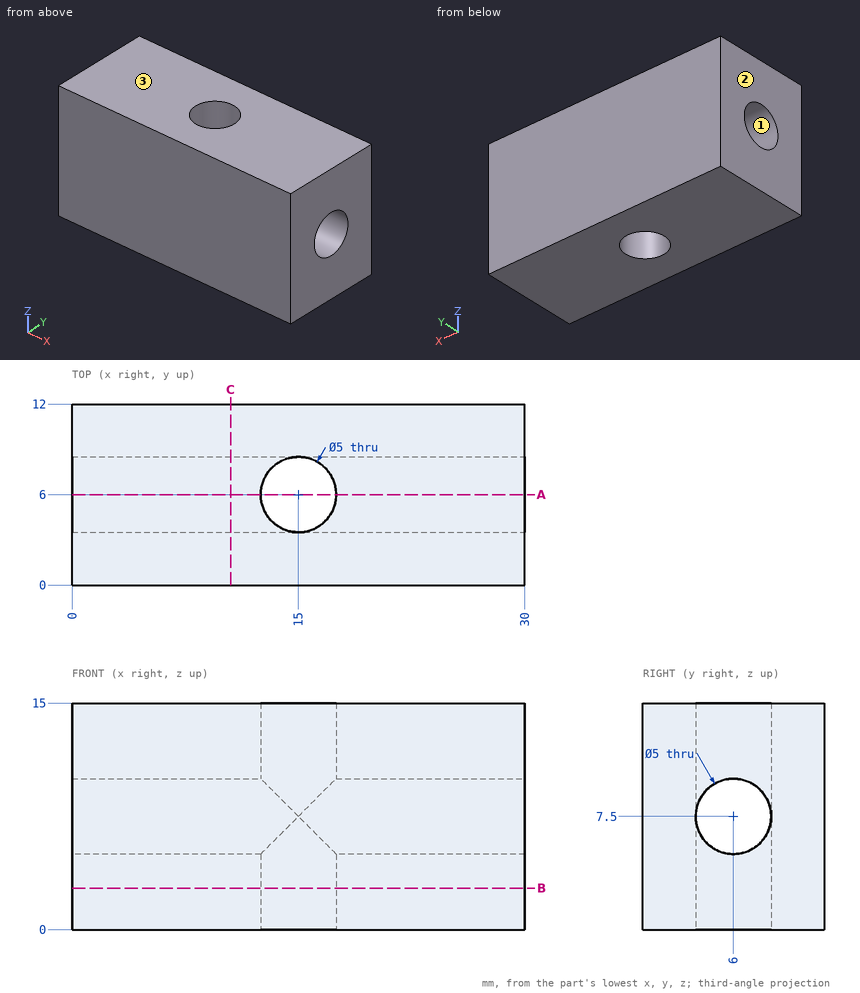
Print and shaded views of the part. All mm, measured from the part's lowest x, y and z. Coordinates: 2 decimals unless noted, no trailing zeros. Order: outer loops, then holes, each group sorted by start corner. A loop starts at its lowest first (then second) coordinate and runs counter-clockwise, first axis right, second up. Notation, with made-up numbers: M 5,24.5 L 28,24.5 A10 cw 28,35.5 Z; hole C -23.5,-19 d5. An arc over 180 degrees is marked long. Write each question's results on one line, items separated by ' | '. Start each with the question number.
Q1. Flat gauge pin, fed straight in: P1, Ø4.5, axis at x = 15, y = 6, coming from the -Z side. Where does the tip first touch, or does it go through?
Q2. Cut at B-B (z = 2.75). List the corners of the cut face in (x, y), then the cut area to 3 significant figures.
Q3. Cut at C-C (x = 10.5). List the corners of the cut face in (y, z).
Q4. Cut at A-A (y = 6). List the corners of the cut face in (x, z), then the cut area to 3 significant figures.
Q5. Pull direction Z, two halves, no side cores. Call the marked faces 1, 2 and 3: +Z half, -Z half, draft (parallel to the pull), parting line (faces both ways), or undercut.
Q6. Drill centre lines: probe 1 along Z at (x, y) = (8.5, 6); probe 2 along Y at (x, z) = (15, 9.75); probe 3 along X at (y, z) = (6, 3.5). Where is each one in solid material? Low to high. Write a range as from..to.
Found:
1) P1: through
2) outline: M 0,0 L 30,0 L 30,12 L 0,12 Z; hole C 15,6 d5 | area: 340 mm²
3) outline: M 0,0 L 12,0 L 12,15 L 0,15 Z; hole C 6,7.5 d5
4) outline: M 0,0 L 12.5,0 L 12.5,5 L 0,5 Z; M 0,10 L 12.5,10 L 12.5,15 L 0,15 Z; M 17.5,0 L 30,0 L 30,5 L 17.5,5 Z; M 17.5,10 L 30,10 L 30,15 L 17.5,15 Z | area: 250 mm²
5) face 1: undercut | face 2: draft | face 3: +Z half
6) probe 1: 0..5, 10..15 | probe 2: 0..3.5, 8.5..12 | probe 3: 0..12.5, 17.5..30
